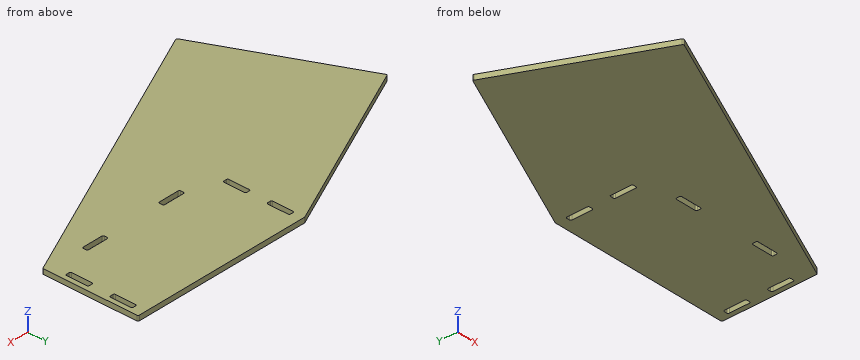
```python
from build123d import *

# Parameters (mm, degrees)
SKETCH1_W           = 416.56
SKETCH1_H           = 219.075
BOSS_EXTRUDE1_DEPTH = 6.35
BOSS_EXTRUDE2_DEPTH = 6.35
FILLET1_R           = 3.175


with BuildPart() as part:
    # Sketch1 → Boss-Extrude1 (new body, symmetric)
    with BuildSketch(Plane.XY):
        with Locations((0, -109.5375)):
            Rectangle(SKETCH1_W, SKETCH1_H)
    extrude(amount=BOSS_EXTRUDE1_DEPTH, both=True)

    # Sketch2 → Boss-Extrude2 (add, symmetric)
    with BuildSketch(Plane.XY):
        Polygon((-221.742, 0), (-682.146355815, -214.690076964), (-509.434106267, -585.072691377), (233.68, -238.552892741), (233.68, 0), (208.28, 0), (208.28, -26.19375), (221.742, -26.19375), (221.742, -83.34375), (208.28, -83.34375), (208.28, -135.73125), (221.742, -135.73125), (221.742, -192.88125), (208.28, -192.88125), (208.28, -219.075), (132.715, -219.075), (132.715, -232.537), (75.565, -232.537), (75.565, -219.075), (-75.565, -219.075), (-75.565, -232.537), (-132.715, -232.537), (-132.715, -219.075), (-208.28, -219.075), (-208.28, -192.88125), (-221.742, -192.88125), (-221.742, -135.73125), (-208.28, -135.73125), (-208.28, -83.34375), (-221.742, -83.34375), (-221.742, -26.19375), (-208.28, -26.19375), (-208.28, 0), align=None)
    extrude(amount=BOSS_EXTRUDE2_DEPTH, both=True)

    # Fillet1
    fillet1_edges = [part.edges().sort_by_distance(p)[0] for p in [
        (-682.146355815, -214.690076964, 0),
        (-509.434106267, -585.072691377, 0),
        (233.68, -238.552892741, 0),
        (233.68, 0, 0),
        (208.28, -26.19375, 0),
        (221.742, -26.19375, 0),
        (221.742, -83.34375, 0),
        (208.28, -83.34375, 0),
        (208.28, -135.73125, 0),
        (221.742, -135.73125, 0),
        (221.742, -192.88125, 0),
        (208.28, -192.88125, 0),
        (132.715, -219.075, 0),
        (132.715, -232.537, 0),
        (75.565, -232.537, 0),
        (75.565, -219.075, 0),
        (-75.565, -219.075, 0),
        (-75.565, -232.537, 0),
        (-132.715, -232.537, 0),
        (-132.715, -219.075, 0),
        (-208.28, -192.88125, 0),
        (-221.742, -192.88125, 0),
        (-221.742, -135.73125, 0),
        (-208.28, -135.73125, 0),
        (-208.28, -83.34375, 0),
        (-221.742, -83.34375, 0),
        (-221.742, -26.19375, 0),
        (-208.28, -26.19375, 0),
        (-221.742, 0, 0),
    ]]
    fillet(fillet1_edges, radius=FILLET1_R)


solid = part.part
```
CAD build for the part. Positions are in the model's coordinates, mm. Round coordinates to 2 decimals unless told otherwise and drop trailing zeros. Order: outer loops, then holes, each group sorted by start corner. A loop starts at its lowest first (then second) coordinate and runs counter-clockwise, first axis right, second up. Notation, with made-up numbers: (8, -24) - (46, -24) arc R10 ccw to (46, -11) - close; hole circle Ø7 at (12.5, 16.5). An arc over 180 degrees is marked (long way). Answer in a Markdown table with one row per item. Add a question column.
(1) Band-saw the part on C-C on x = -91.5. List the corners of the cut face in (y, z) (3 decimals).
(2) Probe L1, parallel to X at y = -54, z = -3; L2, parallel to X at y = -183, z = 1.75; L3, parallel to Y at x = -111, z = -5.5 (3 decimals). List the from-to ranges inside material, lowest first. Write a range as [from, to].
(3) Band-saw the part on B-B on z = 2. Count the separate pieces of the cut face and the enclosed holes in it, and give its area (3 significant figures).
(4) Band-saw the part on A-A on x = 93. List the corners of the cut face in (y, z) (3 decimals).
(5) Drop flat-ended pins along their axis: pin 1 Ø1 at (y, z) = (-289, -5) entering from -X; pin 2 Ø6.5 at (y, z) = (-53, -1) entering from -X; pin 3 Ø6 at (y, z) = (-191, 3.5) entering from -X. Give the stop position or say it passes through.
(6) Band-saw the part on D-D on y = -488. List the corners of the cut face in (x, z), and give its area (3 significant figures).
Data:
| question | item | result |
|---|---|---|
| 1 | outline | (-390.187, -6.35) - (-232.537, -6.35) - (-232.537, 6.35) - (-390.187, 6.35) - close; (-219.075, -6.35) - (0, -6.35) - (0, 6.35) - (-219.075, 6.35) - close |
| 2 | L1 | x = [-337.55, -221.74], [-208.28, 208.28], [221.74, 233.68] |
| 2 | L2 | x = [-614.19, -221.74], [-208.28, 208.28], [221.74, 233.68] |
| 2 | L3 | y = [-399.28, -232.537], [-219.075, 0] |
| 3 | separate pieces | 1 |
| 3 | enclosed holes | 6 |
| 3 | area | 321,000 mm^2 |
| 4 | outline | (-304.153, -6.35) - (-232.537, -6.35) - (-232.537, 6.35) - (-304.153, 6.35) - close; (-219.075, -6.35) - (0, -6.35) - (0, 6.35) - (-219.075, 6.35) - close |
| 5 | pin 1 | stops at x = -647.73 |
| 5 | pin 2 | stops at x = -342.37 |
| 5 | pin 3 | stops at x = -637.78 |
| 6 | outline | (-554.7, -6.35) - (-301.26, -6.35) - (-301.26, 6.35) - (-554.7, 6.35) - close |
| 6 | area | 3,220 mm^2 |
